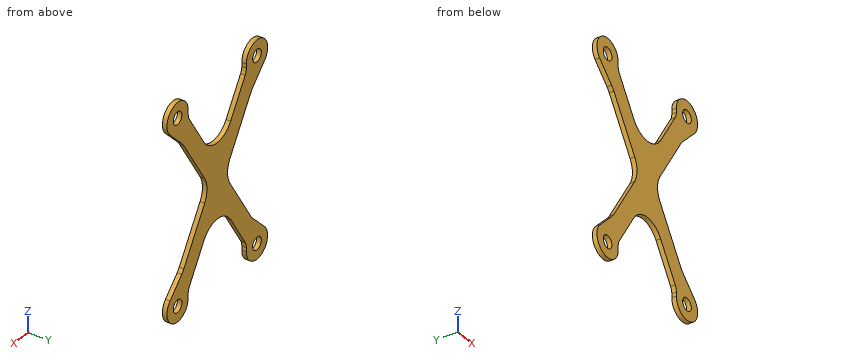
from build123d import *

# Parameters (mm, degrees)
SKETCH1_R           = 2.75
BOSS_EXTRUDE1_DEPTH = 2


with BuildPart() as part:
    # Sketch1 → Boss-Extrude1 (new body)
    with BuildSketch(Plane(origin=(0, 0, 0), x_dir=(1, 0, 0), z_dir=(0, 1, 0))):
        with BuildLine():
            ThreePointArc((-22.650842333, 28.104900787), (-21.901331942, 27.26589175), (-21.250806764, 26.34800342))
            Line((-21.250806764, 26.34800342), (-8.055669308, 5.314170444))
            ThreePointArc((-8.055669308, 5.314170444), (-6.526772689, 0), (-8.055669308, -5.314170444))
            Line((-8.055669308, -5.314170444), (-21.294498712, -26.41765098))
            ThreePointArc((-21.294498712, -26.41765098), (-21.94502389, -27.33553931), (-22.694534281, -28.174548348))
            Line((-22.694534281, -28.174548348), (-30.36172718, -35.841741247))
            ThreePointArc((-30.36172718, -35.841741247), (-27.601418884, -46.577189679), (-18.5, -40.25))
            Line((-18.5, -40.25), (-18.5, -38.455653201))
            ThreePointArc((-18.5, -38.455653201), (-18.305088888, -37.073220282), (-17.735551691, -35.798567979))
            Line((-17.735551691, -35.798567979), (-8.471103381, -21.03048701))
            ThreePointArc((-8.471103381, -21.03048701), (0, -16.344657454), (8.471103381, -21.03048701))
            Line((8.471103381, -21.03048701), (17.735551691, -35.798567979))
            ThreePointArc((17.735551691, -35.798567979), (18.305088888, -37.073220282), (18.5, -38.455653201))
            Line((18.5, -38.455653201), (18.5, -40.25))
            ThreePointArc((18.5, -40.25), (27.833113168, -46.486186844), (30.022970773, -35.477029227))
            Line((30.022970773, -35.477029227), (22.650842334, -28.104900787))
            ThreePointArc((22.650842334, -28.104900787), (21.901331942, -27.26589175), (21.250806764, -26.34800342))
            Line((21.250806764, -26.34800342), (8.055669308, -5.314170444))
            ThreePointArc((8.055669308, -5.314170444), (6.526772689, 0), (8.055669308, 5.314170444))
            Line((8.055669308, 5.314170444), (21.250806764, 26.34800342))
            ThreePointArc((21.250806764, 26.34800342), (21.901331942, 27.26589175), (22.650842333, 28.104900787))
            Line((22.650842333, 28.104900787), (30.022970773, 35.477029227))
            ThreePointArc((30.022970773, 35.477029227), (27.833113168, 46.486186844), (18.5, 40.25))
            Line((18.5, 40.25), (18.5, 38.455653201))
            ThreePointArc((18.5, 38.455653201), (18.305088888, 37.073220282), (17.735551691, 35.798567979))
            Line((17.735551691, 35.798567979), (8.471103381, 21.03048701))
            ThreePointArc((8.471103381, 21.03048701), (0, 16.344657454), (-8.471103381, 21.03048701))
            Line((-8.471103381, 21.03048701), (-17.735551691, 35.798567979))
            ThreePointArc((-17.735551691, 35.798567979), (-18.305088889, 37.073220282), (-18.5, 38.455653201))
            Line((-18.5, 38.455653201), (-18.5, 40.25))
            ThreePointArc((-18.5, 40.25), (-27.833113168, 46.486186844), (-30.022970773, 35.477029227))
            Line((-30.022970773, 35.477029227), (-22.650842333, 28.104900787))
        make_face()
        with Locations(Location((-25.25, -40.25, 0), (0, 0, 270))):
            Circle(SKETCH1_R, mode=Mode.SUBTRACT)
        with Locations(Location((-25.25, 40.25, 0), (0, 0, 270))):
            Circle(SKETCH1_R, mode=Mode.SUBTRACT)
        with Locations(Location((25.25, 40.25, 0), (0, 0, 270))):
            Circle(SKETCH1_R, mode=Mode.SUBTRACT)
        with Locations(Location((25.25, -40.25, 0), (0, 0, 270))):
            Circle(SKETCH1_R, mode=Mode.SUBTRACT)
    extrude(amount=BOSS_EXTRUDE1_DEPTH)


solid = part.part
Build history of the part. All positions in model axes, mm. Round coordinates to 2 decimals unless told otherwise and drop trailing zeros. Write each loop counter-clockwise with the first axis right and the second up, starting at its lowest first coordinate (ties: lowest second). Pieces come first, ordered by that corner, then holes. Notation, with made-up numbers: (49, 42.25) - (92, 42.25) arc R15 cw to (92, 56.25) - close; hole circle Ø11 at (60.5, -21.5). An arc over 180 degrees is marked (long way). One line per question, with ' | ' between items.
1. Band-saw the part on C-C, the plane y = 1.2. Give the number of separate pieces and of enclosed holes in the cut face, and give its area (3 significant figures).
Results are:
separate pieces: 1 | enclosed holes: 4 | area: 1,890 mm^2
2. Band-saw the part on D-D, the plane x = -25.25. Write the cut outline in (y, z).
Results are:
outline: (0, -47) - (2, -47) - (2, -43) - (0, -43) - close; (0, -37.5) - (2, -37.5) - (2, -30.7) - (0, -30.7) - close; (0, 30.73) - (2, 30.73) - (2, 37.5) - (0, 37.5) - close; (0, 43) - (2, 43) - (2, 47) - (0, 47) - close
3. Drill centre lines: line 1 along X through (y, z) = (0.7, 40.25); line 2 along Z through (x, y) = (27, 1.85); line 3 along X through (y, z) = (0.8, -39). Where is each one in solid material? Low to high. Write a range as from..to.
Results are:
line 1: -32..-28, -22.5..-18.5, 18.5..22.5, 28..32 | line 2: -46.77..-42.37, -38.13..-32.45, 32.45..38.13, 42.37..46.77 | line 3: -31.88..-27.7, -22.8..-18.5, 18.5..22.8, 27.7..31.88
4. Band-saw the part on A-A, the plane z = -29.5. Write the cut outline in (x, y).
Results are:
outline: (-24.05, 0) - (-13.78, 0) - (-13.78, 2) - (-24.05, 2) - close; (13.78, 0) - (24.05, 0) - (24.05, 2) - (13.78, 2) - close
5. Band-saw the part on B-B, the plane x = 25.25. Write the cut outline in (y, z).
Results are:
outline: (0, -47) - (2, -47) - (2, -43) - (0, -43) - close; (0, -37.5) - (2, -37.5) - (2, -30.7) - (0, -30.7) - close; (0, 30.7) - (2, 30.7) - (2, 37.5) - (0, 37.5) - close; (0, 43) - (2, 43) - (2, 47) - (0, 47) - close
6. Drop flat-ended pins along their axis: pin 1 Ø7 at (x, z) = (-25.25, -40.25) entering from -Y; pin 2 Ø0.9 at (y, z) = (1, -39.5) entering from +X; pin 3 Ø0.9 at (y, z) = (1, -39.5) entering from -X. Give the stop position or say it passes through.
Results are:
pin 1: y = 0 | pin 2: x = 31.99 | pin 3: x = -31.99
